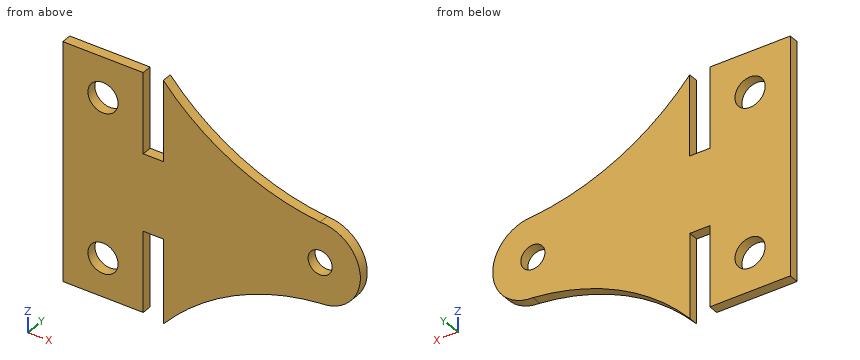
Autodesk Inventor part; units mm, degrees
ref_plane "YZ Plane" through (0, 0, 0) normal (1, 0, 0) x (0, 1, 0)
ref_plane "XZ Plane" through (0, 0, 0) normal (0, 1, 0) x (-1, 0, 0)
ref_plane "XY Plane" through (0, 0, 0) normal (0, 0, 1) x (1, 0, 0)
sketch "Sketch1" plane through (0, 0, 0) normal (0, 1, 0) x (-1, 0, 0)
  arc A0 (0, 6.35) -> (0.0031, -6.35) centre (0, 0) ccw
  line L0 (27.9369, -5.7599) -> (27.9369, -18.4599)
  line L1 (27.94, 6.35) -> (27.94, 19.05)
  line L2 (27.94, 19.05) -> (40.64, 19.05)
  line L3 (40.64, 19.05) -> (40.64, -18.4599)
  line L4 (40.64, -18.4599) -> (27.9369, -18.4599)
  circle A1 centre (0, 0) radius 1.905
  line L5 (27.94, 6.35) -> (24.765, 6.35)
  line L6 (24.765, 6.35) -> (24.765, 19.05)
  line L7 (24.7681, -5.7599) -> (24.7681, -19.05)
  arc A2 (24.7681, -19.05) -> (0.0031, -6.35) centre (-3.7989, -44.2598) ccw
  arc A3 (0, 6.35) -> (24.765, 19.05) centre (-3.802, 44.2598) ccw
  line L8 (24.7681, -5.7599) -> (27.9369, -5.7599)
  point P0 (0, 0)
  dimension "d4" = 27.94
  dimension "d5" = 27.94
  dimension "d6" = 12.7
  dimension "d7" = 12.7
  dimension "d8" = 12.7
  dimension "d19" = 3.81
  dimension "d20" = 3.175
  dimension "d21" = 38.1
  dimension "d22" = 38.1
extrude "Extrusion1" add sketch "Sketch1" along normal blind 1.5875
sketch "Sketch2" plane through (0, 1.5875, 0) normal (0, 1, 0) x (1, 0, 0)
  line L0 (-27.9369, 18.4599) -> (-40.64, 18.4599)
  line L1 (-27.9369, 5.7599) -> (-27.9369, 18.4599)
  line L2 (-40.64, 18.4599) -> (-27.9369, 5.7599)
  line L3 (-40.64, -19.05) -> (-27.94, -19.05)
  line L4 (-27.94, -6.35) -> (0, -6.35)
  line L5 (-40.64, -19.05) -> (-27.94, -6.35)
  line L6 (-27.94, -19.05) -> (-40.64, -6.35)
  line L7 (-27.9369, 18.4599) -> (-40.64, 6.35)
  line L8 (-40.64, 18.4599) -> (-40.64, -19.05)
  point P0 (0, 0)
  point P1 (-34.2884, 12.4049)
  point P2 (-34.29, -12.7)
hole "Hole1" at (-34.2884, 1.5875, -12.4049) at (-34.29, 1.5875, 12.7) direction (0, -1, 0) diameter 4.7625 end through all
properties part number "indexer" material "ABS Plastic"
Work out the finished part from the listing and answer in its coordinate system (mm). Round coordinates to 2 decimals unless told otherwise and drop trailing zeros. Write each loop counter-clockwise with the first axis right and the second up, starting at its lowest first coordinate (ties: lowest second). Pieces come first, ordered by that corner, then holes. Notation, with made-up numbers: (44, -15.5) - (80, -15.5) arc R30 cw to (80, 21.5) - close; hole circle Ø10 at (-31.75, 74). An arc over 180 degrees is marked (long way). Answer in a Markdown table with one row per item. Add a question column.
1. Given pin 1 (0.8 mm diameter, centred on y = 0.5, z = -13.5, fed in from +X); pin 2 (0.5 mm diameter, centred on x = -27, y = 0.5, fed in from -Z); pin 3 (0.8 mm diameter, centred on x = -34, y = 0.5, fed in from -Z), each flat-ended and moving along its own axis, determine where each tip first touches the part or whether it passes through.
2. A cutting plane is placed at C-C, the plane x = -1. Determine the outline of the cut face in (y, z), and give its area (3 significant figures).
3. Find the intervals of material crossed by line 1 along Z through (x, y) = (-34.29, 0.6); line 2 along X through (y, z) = (0.2, -13); line 3 along X through (y, z) = (0.8, 13) (3 decimals), in increasing order. Write a range as from..to.
4. A cutting plane is placed at B-B, the plane z = -14. Determine the outline of the cut face in (x, y), and give its area (3 significant figures).
5. A cutting plane is placed at D-D, the plane y = 1. Count the separate pieces of the cut face and the enclosed holes in it, and give its area (3 significant figures).
Worked out:
| question | item | result |
|---|---|---|
| 1 | pin 1 | x = -18.13 |
| 1 | pin 2 | z = -5.76 |
| 1 | pin 3 | z = -18.46 |
| 2 | outline | (0, -6.46) - (1.59, -6.46) - (1.59, -1.62) - (0, -1.62) - close; (0, 1.62) - (1.59, 1.62) - (1.59, 6.46) - (0, 6.46) - close |
| 2 | area | 15.4 mm^2 |
| 3 | line 1 | -18.46..-14.79, -10.02..10.32, 15.08..19.05 |
| 3 | line 2 | -40.64..-36.59, -31.98..-27.94, -24.77..-17.98 |
| 3 | line 3 | -40.64..-36.652, -31.928..-27.94, -24.765..-17.979 |
| 4 | outline | (-40.64, 0) - (-36.06, 0) - (-36.06, 1.59) - (-40.64, 1.59) - close; (-32.52, 0) - (-27.94, 0) - (-27.94, 1.59) - (-32.52, 1.59) - close; (-24.77, 0) - (-19.35, 0) - (-19.35, 1.59) - (-24.77, 1.59) - close |
| 4 | area | 23.2 mm^2 |
| 5 | separate pieces | 1 |
| 5 | enclosed holes | 3 |
| 5 | area | 1,060 mm^2 |
